from build123d import *

# Parameters (mm, degrees)
F1_DEPTH = 42.926
F2_W     = 20.731261
F2_H     = 19.1265270114
F3_DEPTH = 34.29


with BuildPart() as f1:
    # F0 (on Front) → F1 (new body)
    with BuildSketch(Plane.XZ):
        Polygon((-22.6943474263, -47.376524657), (59.8004348576, -47.376524657), (59.8004348576, -33.1304371357), (-8.4482617676, -33.1304371357), (-8.4482617676, 0), (-58.4752187133, 0), (-58.4752187133, -13.2521744817), (-22.6943474263, -13.2521744817), align=None)
    extrude(amount=F1_DEPTH)

    # F2 (on face) → F3 (join)
    with BuildSketch(Plane.XY.offset(-33.1304371357)):
        with Locations((1.9173687324, -9.5632635057)):
            Rectangle(F2_W, F2_H)
    extrude(amount=F3_DEPTH)


solid = f1.part
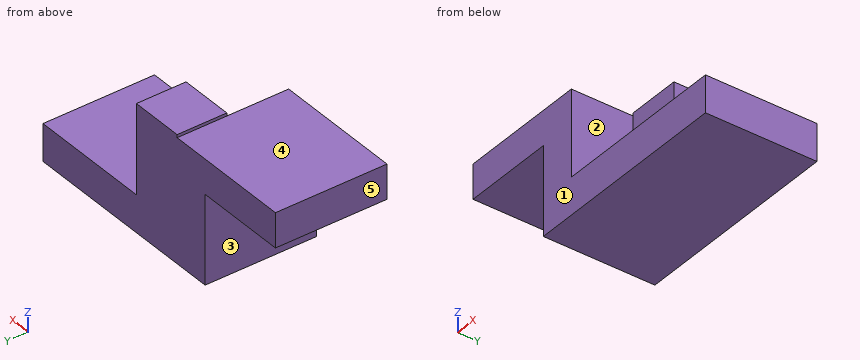
Read the model definition and answer for the solid it produces. Units are mm, in the model's axes. Face numbers are marked on the shaded views. A direction names the side the tool comes from. Coordinates: 2 decimals unless noted, no trailing zeros. Order: outer loops, then holes, each group sorted by start corner. A loop starts at its lowest first (then second) coordinate and runs counter-clockwise, first axis right, second up. Notation, with made-up numbers: M 78,45 L 110,45 A32 ccw 110,76 Z; hole C 81.5,-37.5 d9. An arc over 180 degrees is marked long. Put each result on its own line as item: value. Start each with the question number.
Item 1: Section A-A, the plane y = -24 is taken. Determine the outline of the cut face in (x, z).
Item 2: Section B-B, the plane z = -6 is taken. Determine the outline of the cut face in (x, y).
Item 3: Given pin 1 Ø5 at (x, z) = (-7.5, -29) entering from +Y; pin 2 Ø21.5 at (x, y) = (35.5, -22) entering from +Z; pin 3 Ø1.5 at (x, y) = (-35.5, -6) entering from -Z; pin 4 Ø19 at (y, z) = (-26.5, -23) entering from +X, each flat-ended and moving along its own axis, determine where each tip first touches the part or whether it passes through.
Item 4: Consider probe 1 along Z at (x, y) = (-29, -13); probe 2 along X at (y, z) = (-39, -3.5); probe 3 along Z at (x, y) = (-19, -30). Determine where each line is inside the solid, lowest interval first. Write a range as [from, to].
Item 5: For the marked faces 1, 2, 3, 4 and 5, determine the directions among +Z, -Z, +X, -X, +Y, -Y from which every point of the face is accessible in a straight line to the end or side of a thin tool.
Item 6: Section D-D, the plane y = -9.5 is taken. Determine the outline of the cut face in (x, z), plus the area to 3 significant figures.
Item 7: Section C-C, the plane x = -1.5 is taken. Determine the outline of the cut face in (y, z), plus the area to 3 significant figures.
Computed:
1. outline: M -58.48,-13.25 L -22.69,-13.25 L -22.69,-47.38 L 59.8,-47.38 L 59.8,-33.13 L -8.45,-33.13 L -8.45,0 L -58.48,0 Z
2. outline: M -58.48,-42.93 L -8.45,-42.93 L -8.45,-19.13 L 12.28,-19.13 L 12.28,0 L -58.48,0 Z
3. pin 1: stops at y = 0
3. pin 2: stops at z = -33.13
3. pin 3: stops at z = -13.25
3. pin 4: stops at x = 12.28
4. probe 1: z = [-13.25, 0]
4. probe 2: x = [-58.48, -8.45]
4. probe 3: z = [-47.38, 0]
5. face 1: +Z, -Z, +X, -X, -Y
5. face 2: +Z, +X, -Y
5. face 3: -Z, -X, +Y, -Y
5. face 4: +Z, -X, +Y, -Y
5. face 5: +Z, -Z, -X, +Y, -Y
6. outline: M -58.48,-13.25 L -22.69,-13.25 L -22.69,-47.38 L 59.8,-47.38 L 59.8,-33.13 L 12.28,-33.13 L 12.28,1.16 L -8.45,1.16 L -8.45,0 L -58.48,0 Z
6. area: 2,830 mm2
7. outline: M -42.93,-47.38 L 0,-47.38 L 0,1.16 L -19.13,1.16 L -19.13,-33.13 L -42.93,-33.13 Z
7. area: 1,270 mm2
